Design review of the part built by this model. Coordinates are the model's own, in mm. Give positions to 0.01 mm unless a question says otherwise; leave off trailing zeros. Loops run counter-clockwise (first coordinate to the right, second up) from the corner with the lowest first, then second, coordinate; pieces in that order, holes last. Notation, with made-up numbers: M 47.25,34 L 68.25,34 A26 cw 68.25,62 Z; hole C 6.5,35 d5. An arc over 180 degrees is marked long. Use a Markdown table: item, result. Add a question column.
(1) Add section A-A, the plane x = -27. Give the boundary of the cut face in (y, z).
(2) Insertion check: pin 1 Ø1 at (x, z) = (0.5, 1.5) entering from -Y. The pin has a flat end and moves straight along its axis. Give the tip position at first contact, or say it passes through.
(3) Add section D-D, the plane y = 2. Give the boundary of the cut face in (x, z).
(4) Add section B-B, the plane x = 16.5. Give the boundary of the cut face in (y, z), then the cut area to 3 significant figures.
(5) Add section C-C, the plane z = 30.5. Give the boundary of the cut face in (x, y), then the cut area to 3 significant figures.
(6) For probe 1 along Z at (x, y) = (-29, 2); probe 2 along X at (y, z) = (2.45, 24); probe 3 along X at (y, z) = (2.65, -45), list the stretches that pass through material, from the lowest coordinate up.
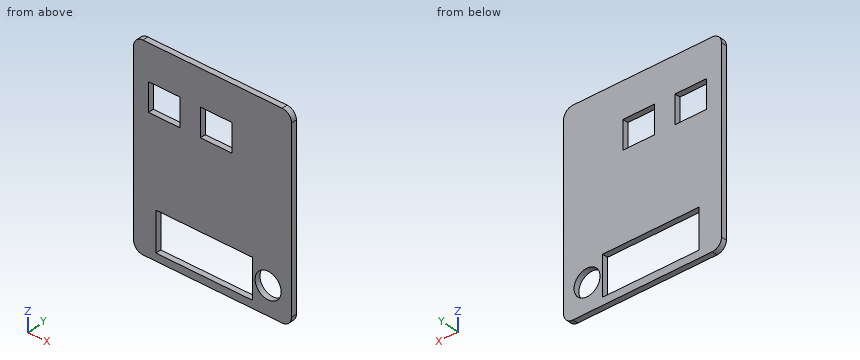
```python
from build123d import *

# Parameters (mm, degrees)
SKETCH1_W           = 85
SKETCH1_H           = 105
BOSS_EXTRUDE1_DEPTH = 3
SKETCH2_W           = 17
SKETCH2_H           = 15
CUT_EXTRUDE1_DEPTH  = 10
FILLET1_R           = 5
SKETCH3_W           = 52
SKETCH3_H           = 21
CUT_EXTRUDE2_DEPTH  = 10
SKETCH4_R           = 7
CUT_EXTRUDE3_DEPTH  = 10


with BuildPart() as part:
    # Sketch1 → Boss-Extrude1 (new body)
    with BuildSketch(Plane(origin=(0, 0, 0), x_dir=(1, 0, 0), z_dir=(0, 1, 0))):
        Rectangle(SKETCH1_W, SKETCH1_H)
    extrude(amount=BOSS_EXTRUDE1_DEPTH)

    # Sketch2 → Cut-Extrude1 (cut)
    with BuildSketch(Plane(origin=(0, 3, 0), x_dir=(1, 0, 0), z_dir=(0, 1, 0))):
        with Locations((-26, -26)):
            Rectangle(SKETCH2_W, SKETCH2_H)
        with Locations((2, -26)):
            Rectangle(SKETCH2_W, SKETCH2_H)
    extrude(amount=-CUT_EXTRUDE1_DEPTH, mode=Mode.SUBTRACT)

    # Fillet1
    fillet1_edges = [part.edges().sort_by_distance(p)[0] for p in [
        (42.5, 1.5, 52.5),
        (-42.5, 1.5, 52.5),
        (-42.5, 1.5, -52.5),
        (42.5, 1.5, -52.5),
    ]]
    fillet(fillet1_edges, radius=FILLET1_R)

    # Sketch3 → Cut-Extrude2 (cut)
    with BuildSketch(Plane(origin=(0, 3, 0), x_dir=(1, 0, 0), z_dir=(0, 1, 0))):
        with Locations((-4.5, 38)):
            Rectangle(SKETCH3_W, SKETCH3_H)
    extrude(amount=-CUT_EXTRUDE2_DEPTH, mode=Mode.SUBTRACT)

    # Sketch4 → Cut-Extrude3 (cut)
    with BuildSketch(Plane(origin=(0, 3, 0), x_dir=(1, 0, 0), z_dir=(0, 1, 0))):
        with Locations(Location((29.897939867, 37.565399996, 0), (0, 0, 270))):
            Circle(SKETCH4_R)
    extrude(amount=-CUT_EXTRUDE3_DEPTH, mode=Mode.SUBTRACT)


solid = part.part
```
Established:
| question | item | result |
|---|---|---|
| 1 | outline | M 0,-52.5 L 3,-52.5 L 3,-48.5 L 0,-48.5 Z; M 0,-27.5 L 3,-27.5 L 3,18.5 L 0,18.5 Z; M 0,33.5 L 3,33.5 L 3,52.5 L 0,52.5 Z |
| 2 | pin 1 | y = 0 |
| 3 | outline | M -42.5,-47.5 A5 ccw -37.5,-52.5 L 37.5,-52.5 A5 ccw 42.5,-47.5 L 42.5,47.5 A5 ccw 37.5,52.5 L -37.5,52.5 A5 ccw -42.5,47.5 Z; hole M -34.5,18.5 L -17.5,18.5 L -17.5,33.5 L -34.5,33.5 Z; hole M -30.5,-48.5 L 21.5,-48.5 L 21.5,-27.5 L -30.5,-27.5 Z; hole M -6.5,18.5 L 10.5,18.5 L 10.5,33.5 L -6.5,33.5 Z; hole C 29.9,-37.57 d14 |
| 4 | outline | M 0,-52.5 L 3,-52.5 L 3,-48.5 L 0,-48.5 Z; M 0,-27.5 L 3,-27.5 L 3,52.5 L 0,52.5 Z |
| 4 | area | 252 mm^2 |
| 5 | outline | M -42.5,0 L -34.5,0 L -34.5,3 L -42.5,3 Z; M -17.5,0 L -6.5,0 L -6.5,3 L -17.5,3 Z; M 10.5,0 L 42.5,0 L 42.5,3 L 10.5,3 Z |
| 5 | area | 153 mm^2 |
| 6 | probe 1 | -52.5 to -48.5, -27.5 to 18.5, 33.5 to 52.5 |
| 6 | probe 2 | -42.5 to -34.5, -17.5 to -6.5, 10.5 to 42.5 |
| 6 | probe 3 | -42.5 to -30.5, 21.5 to 42.5 |
